Source: CAD feature listing. Evaluate the final solid. Frame: model axes, mm. A direction names the side the tool comes from. Coordinates: 2 decimals unless noted, no trailing zeros. Loops run counter-clockwise (first coordinate to the right, second up) from the corner with the lowest first, then second, coordinate; pieces in that order, holes last.
Item 1: Reachability of faces 5 (the flat face through (159, -140, 5)), 6 (the flat face through (153, -70, -2)), 7 (the flat face through (243, -69, 5)), 8 (the flat face through (71.616, -35.49, 4.93)) from +Z, -Z, +X, -X, +Y, -Y: full face, straight path, thin tool, end or side. Return the list, or none.
Item 2: Pin query (flat end, axial travel): pin 1 Ø1 at (y, z) = (-85.5, -2) entering from -X; pin 2 Ø1.2 at (x, z) = (9, -1) entering from -Y; pin 3 Ø8 at (x, y) = (160, -97.5) entering from +Z. Return the tip coordinate at first contact, or that it passes through.
Item 3: Section query B-B, the plane y = -105.5. Return the cut outline in (x, z), then the cut area to 3 significant figures.
Item 4: Pull-direction query (X, two-part tool) for faces 1 (the flat face through (247, -69, 5)), 2 (the flat face through (146, 0, -1)), 3 (the flat face through (160, -67, 0)), 4 (the flat face through (69, -115, -1)); classes: +X half, -X half, draft (parallel to the pull), parting line (faces both ways), or undercut.
Item 5: Section query A-A, the plane z = 3. Return the cut outline in (x, y).
Item 6: Section query D-D, the plane x = 254. Return the cut outline in (y, z).
Item 7: Section query C-C, the plane x = 108. Return the cut outline in (y, z).
Item 8: Line query: probe 1 along Y at (x, z) = (199.5, -2.25); probe 2 along X at (y, z) = (-131, 8); probe 3 along Y at (x, z) = (225.5, 4). Output: solid intervals per line, ascending.
```python
from build123d import *

# Parameters (mm, degrees)
BOSS_EXTRUDE1_DEPTH = 4
BOSS_EXTRUDE2_DEPTH = 10


with BuildPart() as part:
    # Sketch1 → Boss-Extrude1 (new body)
    with BuildSketch(Plane.XY):
        with BuildLine():
            Line((270, 0), (0, 0))
            Line((0, 0), (0, -21))
            Line((0, -21), (30, -21))
            ThreePointArc((30, -21), (64.648232278, -35.351767722), (79, -70))
            Line((79, -70), (230, -70))
            Line((230, -70), (270, -70))
            Line((270, -70), (270, 0))
        make_face()
        Polygon((270, -159), (270, -70), (230, -70), (230, -71), (69, -71), (69, -159), align=None)
    extrude(amount=-BOSS_EXTRUDE1_DEPTH)

    # Sketch2 → Boss-Extrude2 (add)
    with BuildSketch(Plane.XY):
        Polygon((247, 0), (247, -140), (69, -140), (69, -136), (243, -136), (243, 0), align=None)
        Polygon((115, -70), (27, 0), (33.425459564, 0), (117.490094263, -66.869595783), (121.425459564, -70), align=None)
    extrude(amount=BOSS_EXTRUDE2_DEPTH)


solid = part.part
```
Verdict:
1. face 5: +Z, +X, -X, -Y
1. face 6: +Z, -Z, -X
1. face 7: +Z, +Y
1. face 8: +Z, -X
2. pin 1: stops at x = 69
2. pin 2: stops at y = -21
2. pin 3: stops at z = 0
3. outline: (69, -4) - (270, -4) - (270, 0) - (247, 0) - (247, 10) - (243, 10) - (243, 0) - (69, 0) - close
3. area: 844 mm2
4. face 1: +X half
4. face 2: draft
4. face 3: undercut
4. face 4: -X half
5. outline: (27, 0) - (115, -70) - (121.43, -70) - (33.43, 0) - close; (69, -140) - (247, -140) - (247, 0) - (243, 0) - (243, -136) - (69, -136) - close
6. outline: (-159, -4) - (0, -4) - (0, 0) - (-159, 0) - close
7. outline: (-159, -4) - (-71, -4) - (-71, 0) - (-136, 0) - (-136, 10) - (-140, 10) - (-140, 0) - (-159, 0) - close; (-70, -4) - (0, -4) - (0, 0) - (-59.32, 0) - (-59.32, 10) - (-64.43, 10) - (-64.43, 0) - (-70, 0) - close
8. probe 1: y = -159 to -71, -70 to 0
8. probe 2: x = 243 to 247
8. probe 3: y = -140 to -136
